The listing builds one solid part. Answer for the finished solid, in the listing's coordinates (mm). A direction names the side the tool comes from. Give positions to 0.01 mm unless a question says otherwise; leave off trailing zeros. Loops run counter-clockwise (first coordinate to the right, second up) from the corner with the lowest first, then second, coordinate; pieces in that order, holes last.
Item 1: Each of these flat-tipped pins is pushed along its axis until it touches: pin 1 Ø0.6 at (x, z) = (-2, 2) entering from +Y; pin 2 Ø1 at (x, z) = (-2, 1) entering from -Y. Where does it stop, or does it pass through?
Item 2: Consider line 1 along Z through (x, y) = (-1.8, 4.7); line 2 along X through (y, z) = (2.75, 0.15); line 3 along Y through (x, z) = (-0.2, -0.1). Determine where each line is inside the solid, lowest interval first.
Item 3: Section B-B, the plane z = 1.65 is taken. Give the vertices of the cut face in (x, y).
Item 4: Section A-A, the plane y = 4.3 is taken. Give the vertices of the cut face in (x, z).
Item 5: Section D-D, the plane y = 2.25 is taken. Give the vertices of the cut face in (x, z), and give its area (3 significant figures).
Item 6: Section C-C, the plane x = -1.3 is taken. Give the vertices of the cut face in (y, z), and give its area (3 significant figures).
Item 7: The mould has two halves that part along Y. Classify faces 1 (the face through (1, 0, -1)), 2 (the face through (-2.2, 0.3, -0.5)), 3 (the face through (-2, 3, 1)), 4 (the face through (-1, 2.5, 1.2)): pulls with the +Y half, pulls with the -Y half, needs draft (parallel to the pull), parting line crosses it, or undercut.
Item 8: A tool of negligible diameter and unlimited length cuts with its end or side. For faces 5 (the face through (1, 2, 3)), 6 (the face through (-2, 2.5, -0.5)), 7 (the face through (-1.5, 0.5, 1.3)), 8 (the face through (-3, 2, -1)), 9 (the face through (-1.5, 4.5, 1.3)), from which of +Z, -Z, +X, -X, +Y, -Y can it reach the whole face along a straight path? Write none if from no direction.
from build123d import *

# Parameters (mm, degrees)
SKETCH1_W           = 6
SKETCH1_H           = 6
BOSS_EXTRUDE1_DEPTH = 5
SKETCH2_W           = 3.5
SKETCH2_H           = 1
CUT_EXTRUDE1_DEPTH  = 2
CUT_EXTRUDE2_DEPTH  = 3.5


with BuildPart() as part:
    # Sketch1 → Boss-Extrude1 (new body)
    with BuildSketch(Plane(origin=(0, 0, 0), x_dir=(1, 0, 0), z_dir=(0, 1, 0))):
        Rectangle(SKETCH1_W, SKETCH1_H)
    extrude(amount=BOSS_EXTRUDE1_DEPTH)

    # Sketch2 → Cut-Extrude1 (cut)
    with BuildSketch(Plane.ZY.offset(3)):
        with Locations((1.25, 2.5)):
            Rectangle(SKETCH2_W, SKETCH2_H)
    extrude(amount=-CUT_EXTRUDE1_DEPTH, mode=Mode.SUBTRACT)

    # Sketch3 → Cut-Extrude2 (cut)
    with BuildSketch(Plane.XY.offset(3)):
        Polygon((-3, 5), (-3, 4), (0, 5), align=None)
        Polygon((-3, 0), (0, 0), (-3, 1), align=None)
    extrude(amount=-CUT_EXTRUDE2_DEPTH, mode=Mode.SUBTRACT)


solid = part.part
Worked answers:
1. pin 1: stops at y = 4.43
1. pin 2: stops at y = 0.5
2. line 1: z = -3 to -0.5
2. line 2: x = -1 to 3
2. line 3: y = 0.07 to 4.93
3. outline: (-3, 1) - (0, 0) - (3, 0) - (3, 5) - (0, 5) - (-3, 4) - (-3, 3) - (-1, 3) - (-1, 2) - (-3, 2) - close
4. outline: (-3, -3) - (3, -3) - (3, 3) - (-2.1, 3) - (-2.1, -0.5) - (-3, -0.5) - close
5. outline: (-3, -3) - (3, -3) - (3, 3) - (-1, 3) - (-1, -0.5) - (-3, -0.5) - close
5. area: 29.0 mm2
6. outline: (0, -3) - (5, -3) - (5, -0.5) - (4.57, -0.5) - (4.57, 3) - (3, 3) - (3, -0.5) - (2, -0.5) - (2, 3) - (0.43, 3) - (0.43, -0.5) - (0, -0.5) - close
6. area: 23.5 mm2
7. face 1: pulls with the -Y half
7. face 2: needs draft
7. face 3: undercut
7. face 4: undercut
8. face 5: +Z, +X, -X, +Y, -Y
8. face 6: +Z, -X
8. face 7: +Z, -X, -Y
8. face 8: +Z, -Z, -X, +Y, -Y
8. face 9: +Z, -X, +Y
